Geometry: final body of the model. Coordinates: model frame, mm. Give positions to 0.01 mm unless a question says otherwise; leave off trailing zeros. Loops run counter-clockwise (first coordinate to the right, second up) from the corner with the lowest first, then second, coordinate; pieces in that order, holes last. Notation, with made-up numbers: (10.25, 89.5) - (36.25, 89.5) arc R19 cw to (36.25, 116.5) - close; hole circle Ø3 at (57, 21). An arc over 180 degrees is marked (long way). Answer in a Markdown table with one row per item.
from build123d import *

# Parameters (mm, degrees)
F0_R     = 10.3520416824
F0_R_2   = 15.1016918028
F1_DEPTH = 12.5


with BuildPart() as f1:
    # F0 (on Front) → F1 (new body, symmetric)
    with BuildSketch(Plane.XZ):
        Polygon((-315.6363590755, 402.8576135222), (-315.6363590755, -445.1646387913), (-237.9194677537, -445.1646387913), (-202.4295538493, 294.5199684009), (-202.4295538493, -526.0605984591), (227.1852354976, -526.0605984591), (206.6384547892, 294.5199684009), (243.9962564237, -445.1646387913), (315.6363590755, -448.601916045), (315.6363590755, 386.046592596), (197.2990004611, 449.5548381291), (53.1655277069, 498.2233074495), (0, 496.8920787035), (-14.4139876592, 496.531162231), (-50.8757645807, 495.6181840727), (-178.146982003, 449.5548381291), align=None)
        with Locations((35.982593894, -126.2090504169)):
            Circle(F0_R, mode=Mode.SUBTRACT)
        with Locations((0, 92.1598300338)):
            Circle(F0_R_2, mode=Mode.SUBTRACT)
        with BuildLine():
            Line((-14.4139876592, 514.4077504381), (-14.4139876592, 496.531162231))
            Line((-14.4139876592, 496.531162231), (0, 496.8920787035))
            Line((0, 496.8920787035), (0, 509.4077504381))
            ThreePointArc((0, 509.4077504381), (26.5864663022, 573.3541076459), (-37.4994765184, 547.1058939281))
            Line((-37.4994765184, 547.1058939281), (-32.499546316, 547.0794747961))
            ThreePointArc((-32.499546316, 547.0794747961), (23.0416041286, 569.8279266848), (0, 514.4077504381))
            Line((0, 514.4077504381), (-14.4139876592, 514.4077504381))
        make_face()
    extrude(amount=F1_DEPTH, both=True)


solid = f1.part
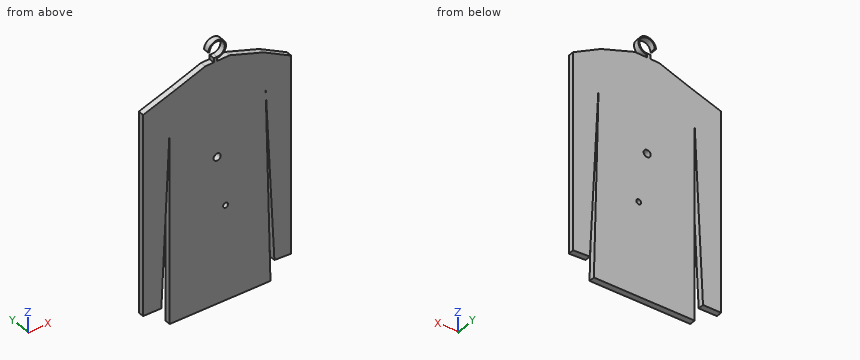
Q1. Material intervals for line 1 along Z through (x, y) = (-1.5, -7); line 2 along Z through (x, y) = (11.5, 8.75); line 3 along Z through (x, y) = (13.5, 4.25), sorted ascending.
Check values:
| item | result |
|---|---|
| line 1 | -526.06 to 77.13, 107.19 to 514.41, 579.37 to 584.38 |
| line 2 | -526.06 to 82.37, 101.95 to 497.18, 511.21 to 516.51, 577.31 to 582.6 |
| line 3 | -526.06 to 85.39, 98.93 to 497.23, 511.92 to 517.34, 576.47 to 581.89 |
Q2. Cut plane A-A (z = -354). Output: boundary loops of the cut face in (x, y).
Check values:
| item | result |
|---|---|
| outline | (-315.64, -12.5) - (-233.55, -12.5) - (-233.55, 12.5) - (-315.64, 12.5) - close; (-202.43, -12.5) - (222.88, -12.5) - (222.88, 12.5) - (-202.43, 12.5) - close; (239.39, -12.5) - (315.64, -12.5) - (315.64, 12.5) - (239.39, 12.5) - close |
Q3. Cut plane D-D (x = 264). Output: boundary loops of the cut face in (y, z).
Check values:
| item | result |
|---|---|
| outline | (-12.5, -446.12) - (12.5, -446.12) - (12.5, 413.76) - (-12.5, 413.76) - close |
Q4. Cut plane B-B (y = 7). Output: boundary loops of the cut face in (x, z), and give its area (3 significant figures).
Check values:
| item | result |
|---|---|
| outline | (-315.64, -445.16) - (-237.92, -445.16) - (-202.43, 294.52) - (-202.43, -526.06) - (227.19, -526.06) - (206.64, 294.52) - (244, -445.16) - (315.64, -448.6) - (315.64, 386.05) - (197.3, 449.55) - (53.17, 498.22) - (0, 496.89) - (0, 509.41) arc R37.5 ccw (long way) to (-37.5, 547.11) - (-32.5, 547.08) arc R32.5 cw (long way) to (0, 514.41) - (-14.41, 514.41) - (-14.41, 496.53) - (-50.88, 495.62) - (-178.15, 449.55) - (-315.64, 402.86) - close; hole circle Ø30.2 at (0, 92.16); hole circle Ø20.7 at (35.98, -126.21) |
| area | 584,000 mm² |
Q5. Cut plane C-C (z = -222.5). Output: boundary loops of the cut face in (x, y).
Check values:
| item | result |
|---|---|
| outline | (-315.64, -12.5) - (-227.24, -12.5) - (-227.24, 12.5) - (-315.64, 12.5) - close; (-202.43, -12.5) - (219.58, -12.5) - (219.58, 12.5) - (-202.43, 12.5) - close; (232.75, -12.5) - (315.64, -12.5) - (315.64, 12.5) - (232.75, 12.5) - close |
Q6. First-contact query: pin 1 (14.5 mm diameter, centred on y = -2, z = 507, fed in from -X); pin 2 (7 mm diameter, centred on x = -8, y = 3, fed in from +Z); pin 3 (6 mm diameter, centred on x = 61.5, y = -2.5, fed in from +Z); pin 4 (16.5 mm diameter, centred on x = 35.98, z = -126.21, fed in from +Y). Flat tips, straight axial feed; report the tip coordinate or a pass-through.
Check values:
| item | result |
|---|---|
| pin 1 | x = -14.41 |
| pin 2 | z = 584.14 |
| pin 3 | z = 496.42 |
| pin 4 | through |
